Geometry: final body of the model. Coordinates: model frame, mm. Coordinates: 2 decimals unless noted, no trailing zeros. Loops run counter-clockwise (first coordinate to the right, second up) from the corner with the lowest first, then second, coordinate; pieces in that order, holes last. Notation, with made-up numbers: (7.5, 49) -> (29.5, 49) arc R14 cw to (29.5, 54) -> close; hole circle Ø11 at (61.25, 23.5). An arc over 180 degrees is marked (long way). One line per item, written item: value. Start each with the question number.
Item 1: Ray query, probe 1 along Y at (x, z) = (60, 1); probe 2 along Y at (x, z) = (59, 1.8); probe 3 along X at (y, z) = (-70, 0.95). Return the intervals inside material, ascending. Write a range as from..to.
Item 2: Section query B-B on z = 2.1. Return loops of the section in (x, y).
Item 3: Contact query for a flat-ended pin moving along its axis: pin 1 Ø3.5 at (x, y) = (-60, 15) entering from +Z. Output: stop coordinate, or through.
Item 4: Section query A-A on x = -26. Return loops of the section in (y, z).
from build123d import *

# Parameters (mm, degrees)
ESQUISSE1_W             = 148
ESQUISSE1_H             = 330
BOSS_EXTRU_1_DEPTH      = 3
ENL_V_MAT_EXTRU_2_REACH = 182.859
ESQUISSE3_R             = 2.2
ENL_V_MAT_EXTRU_3_REACH = 182.859
ESQUISSE4_W             = 148
ESQUISSE4_H             = 10
ENL_V_MAT_EXTRU_4_REACH = 182.859


with BuildPart() as part:
    # Esquisse1 → Boss.-Extru.1 (new body)
    with BuildSketch(Plane.XY):
        Rectangle(ESQUISSE1_W, ESQUISSE1_H)
    extrude(amount=BOSS_EXTRU_1_DEPTH)

    # Esquisse3 → Enl_v. mat.-Extru.2 (cut, up to next)
    with BuildSketch(Plane.XY.offset(3), mode=Mode.PRIVATE) as enl_v_mat_extru_2_sk1:
        with Locations((60, -75)):
            Circle(ESQUISSE3_R)
    enl_v_mat_extru_2_tool1 = extrude(enl_v_mat_extru_2_sk1.sketch, amount=-ENL_V_MAT_EXTRU_2_REACH, mode=Mode.PRIVATE) & part.part
    # Esquisse3 → Enl_v. mat.-Extru.2 (cut, up to next)
    with BuildSketch(Plane.XY.offset(3), mode=Mode.PRIVATE) as enl_v_mat_extru_2_sk2:
        with Locations((60, 15)):
            Circle(ESQUISSE3_R)
    enl_v_mat_extru_2_tool2 = extrude(enl_v_mat_extru_2_sk2.sketch, amount=-ENL_V_MAT_EXTRU_2_REACH, mode=Mode.PRIVATE) & part.part
    enl_v_mat_extru_2_1 = enl_v_mat_extru_2_tool1.solids().sort_by_distance((60, -75, 3))[0]
    add(enl_v_mat_extru_2_1, mode=Mode.SUBTRACT)
    enl_v_mat_extru_2_2 = enl_v_mat_extru_2_tool2.solids().sort_by_distance((60, 15, 3))[0]
    add(enl_v_mat_extru_2_2, mode=Mode.SUBTRACT)
    enl_v_mat_extru_2 = enl_v_mat_extru_2_1 + enl_v_mat_extru_2_2  # Enl_v. mat.-Extru.2 as one shape, for the pattern or mirror that repeats it

    # Esquisse4 → Enl_v. mat.-Extru.3 (cut, up to next)
    with BuildSketch(Plane.XY.offset(3), mode=Mode.PRIVATE) as enl_v_mat_extru_3_sk1:
        with Locations((0, 160)):
            Rectangle(ESQUISSE4_W, ESQUISSE4_H)
    enl_v_mat_extru_3_tool1 = extrude(enl_v_mat_extru_3_sk1.sketch, amount=-ENL_V_MAT_EXTRU_3_REACH, mode=Mode.PRIVATE) & part.part
    add(enl_v_mat_extru_3_tool1.solids().sort_by_distance((0, 160, 3))[0], mode=Mode.SUBTRACT)

    # Sym_trie1: Enl_v. mat.-Extru.2 across plane
    add(enl_v_mat_extru_2.mirror(Plane(origin=(0, 0, 0), x_dir=(0, 0, 1), z_dir=(1, 0, 0))), mode=Mode.SUBTRACT)

    # Esquisse5 → Enl_v. mat.-Extru.4 (cut, up to next)
    with BuildSketch(Plane(origin=(0, 0, 0), x_dir=(-1, 0, 0), z_dir=(0, 0, -1)), mode=Mode.PRIVATE) as enl_v_mat_extru_4_sk1:
        Polygon((17, -77), (37, -77), (41, -73), (41, -63), (41, -53), (36, -49), (18, -49), (13, -53), (13, -63), (13, -73), align=None)
    enl_v_mat_extru_4_tool1 = extrude(enl_v_mat_extru_4_sk1.sketch, amount=-ENL_V_MAT_EXTRU_4_REACH, mode=Mode.PRIVATE) & part.part
    add(enl_v_mat_extru_4_tool1.solids().sort_by_distance((-27, -63.067736, 0))[0], mode=Mode.SUBTRACT)


solid = part.part
Reply:
1. probe 1: y = -165..-77.2, -72.8..12.8, 17.2..155
1. probe 2: y = -165..-76.96, -73.04..13.04, 16.96..155
1. probe 3: x = -74..-41, -13..74
2. outline: (-74, -165) -> (74, -165) -> (74, 155) -> (-74, 155) -> close; hole circle Ø4.4 at (-60, -75); hole circle Ø4.4 at (-60, 15); hole (-41, -73) -> (-37, -77) -> (-17, -77) -> (-13, -73) -> (-13, -53) -> (-18, -49) -> (-36, -49) -> (-41, -53) -> close; hole circle Ø4.4 at (60, -75); hole circle Ø4.4 at (60, 15)
3. pin 1: passes through
4. outline: (-165, 0) -> (-77, 0) -> (-77, 3) -> (-165, 3) -> close; (-49, 0) -> (155, 0) -> (155, 3) -> (-49, 3) -> close
